from build123d import *

# Parameters (mm, degrees)
F1_DEPTH = 5
F9_R     = 1.5
F12_R    = 1.5
F15_R    = 1.5
F18_R    = 1.5
F21_R    = 1.5
F24_R    = 1.5
F28_R    = 1.5
F32_R    = 1.5
F31_R    = 1.5
F36_R    = 1.5


with BuildPart() as f1:
    # F0 (on Top) → F1 (new body, symmetric)
    with BuildSketch(Plane.XY):
        Polygon((-5, -5), (5, -5), (5, -1.9098300548), (0, 0), (-5, -1.9098300548), align=None)
        Polygon((0, 0), (5, -1.9098300548), (5, 1.9098300548), align=None)
        Polygon((-5, 1.9098300548), (-5, -1.9098300548), (0, 0), align=None)
        Polygon((0, 0), (5, 1.9098300548), (5, 5), (-5, 5), (-5, 1.9098300548), align=None)
    extrude(amount=F1_DEPTH, both=True)

    # F10: sweep along a path in F3
    with BuildLine(Plane(origin=(0, 0, 0), x_dir=(-0.7071067812, 0.7071067812, 0), z_dir=(0.7071067812, 0.7071067812, 0))) as f10_path:
        Line((-70.710678, 50), (70.710678, -50))
    # F9 (on line) → F10 (sweep)
    with BuildSketch(Plane(origin=(49.9999999161, -49.9999999161, 50), x_dir=(-0.8164965812, -0.4082482899, 0.4082482906), z_dir=(-0.5773502689, 0.5773502689, -0.5773502698))):
        Circle(F9_R)
    sweep(path=f10_path.line)

    # F13: sweep along a path in F3
    with BuildLine(Plane(origin=(0, 0, 0), x_dir=(-0.7071067812, 0.7071067812, 0), z_dir=(0.7071067812, 0.7071067812, 0))) as f13_path:
        Line((-70.710678, -50), (70.710678, 50))
    # F12 (on line) → F13 (sweep)
    with BuildSketch(Plane(origin=(49.9999999161, -49.9999999161, -50), x_dir=(-0.8164965812, -0.4082482899, -0.4082482906), z_dir=(-0.5773502689, 0.5773502689, 0.5773502698))):
        Circle(F12_R)
    sweep(path=f13_path.line)

    # F16: sweep along a path in F5
    with BuildLine(Plane(origin=(0, 0, 0), x_dir=(0.7071067812, 0.7071067812, 0), z_dir=(0.7071067812, -0.7071067812, 0))) as f16_path:
        Line((70.710678, -50), (-70.710678, 50))
    # F15 (on line) → F16 (sweep)
    with BuildSketch(Plane(origin=(-49.9999999161, -49.9999999161, 50), x_dir=(0.8164965812, -0.4082482899, 0.4082482906), z_dir=(-0.5773502689, -0.5773502689, 0.5773502698))):
        Circle(F15_R)
    sweep(path=f16_path.line)

    # F19: sweep along a path in F5
    with BuildLine(Plane(origin=(0, 0, 0), x_dir=(0.7071067812, 0.7071067812, 0), z_dir=(0.7071067812, -0.7071067812, 0))) as f19_path:
        Line((70.710678, 50), (-70.710678, -50))
    # F18 (on line) → F19 (sweep)
    with BuildSketch(Plane(origin=(-49.9999999161, -49.9999999161, -50), x_dir=(0.8164965812, -0.4082482899, -0.4082482906), z_dir=(-0.5773502689, -0.5773502689, -0.5773502698))):
        Circle(F18_R)
    sweep(path=f19_path.line)

    # F22: sweep along a path in F7
    with BuildLine(Plane.YZ) as f22_path:
        Line((-80.9016994, -30.9016994), (80.9016994, 30.9016994))
    # F21 (on line) → F22 (sweep)
    with BuildSketch(Plane(origin=(0, -80.9016994, -30.9016994), x_dir=(-1, 0, 0), z_dir=(0, 0.9341723591, 0.3568220895))):
        Circle(F21_R)
    sweep(path=f22_path.line)

    # F25: sweep along a path in F7
    with BuildLine(Plane.YZ) as f25_path:
        Line((-80.9016994, 30.9016994), (80.9016994, -30.9016994))
    # F24 (on line) → F25 (sweep)
    with BuildSketch(Plane(origin=(0, 80.9016994, -30.9016994), x_dir=(-1, 0, 0), z_dir=(0, 0.9341723591, -0.3568220895))):
        Circle(F24_R)
    sweep(path=f25_path.line)

    # F29: sweep along a path in F0
    with BuildLine(Plane.XY) as f29_path:
        Line((80.9016994, 30.9016994), (-80.9016994, -30.9016994))
    # F28 (on line) → F29 (sweep)
    with BuildSketch(Plane(origin=(80.9016994, 30.9016994, 0), x_dir=(0.3568220895, -0.9341723591, 0), z_dir=(-0.9341723591, -0.3568220895, 0))):
        Circle(F28_R)
    sweep(path=f29_path.line)

    # F33: sweep along a path in F0
    with BuildLine(Plane.XY) as f33_path:
        Line((-80.9016994, 30.9016994), (80.9016994, -30.9016994))
    # F32 (on line) → F33 (sweep)
    with BuildSketch(Plane(origin=(80.9016994, -30.9016994, 0), x_dir=(0.3568220895, 0.9341723591, 0), z_dir=(0.9341723591, -0.3568220895, 0))):
        Circle(F32_R)
    sweep(path=f33_path.line)

    # F34: sweep along a path in F6
    with BuildLine(Plane.XZ) as f34_path:
        Line((-30.9016994, -80.9016994), (30.9016994, 80.9016994))
    # F31 (on line) → F34 (sweep)
    with BuildSketch(Plane(origin=(30.9016994, 0, 80.9016994), x_dir=(0.9341723591, 0, -0.3568220895), z_dir=(0.3568220895, 0, 0.9341723591))):
        Circle(F31_R)
    sweep(path=f34_path.line)

    # F37: sweep along a path in F6
    with BuildLine(Plane.XZ) as f37_path:
        Line((-30.9016994, 80.9016994), (30.9016994, -80.9016994))
    # F36 (on line) → F37 (sweep)
    with BuildSketch(Plane(origin=(-30.9016994, 0, 80.9016994), x_dir=(0.9341723591, 0, 0.3568220895), z_dir=(0.3568220895, 0, -0.9341723591))):
        Circle(F36_R)
    sweep(path=f37_path.line)


solid = f1.part
The model under review builds one solid part; all positions refer to its coordinate system, in mm. Round coordinates to 2 decimals unless told otherwise and drop trailing zeros. Return JSON: item names as keys, results as strings.
1. Insertion check: P1, Ø12, axis at y = 63, z = 29, coming from the -X side; P2, Ø8, axis at y = -34, z = 42, coming from the -X side; P3, Ø12, axis at x = -13, z = 4, coming from the -Y side. Each pin has a flat end and moves straight along its axis. Give the tip position at first contact, or say it passes through.
Answer block:
{"P1": "stops at x = -1.5", "P2": "passes through", "P3": "stops at y = -11.79"}
2. Take a section at A-A (x = -11). State how many separate pieces and enclosed holes the cut face has, then the cut area to 3 significant figures.
Answer block:
{"separate pieces": "8", "enclosed holes": "0", "area": "104 mm²"}
3. For L1, parallel to Y at x = -14.5, z = 14.5; L2, parallel to X at y = -15, z = 14; L3, parallel to Y at x = 15, z = 41, list the stretches that pass through material, from the lowest coordinate up. Write a range as [from, to].
Answer block:
{"L1": "y = [-16.34, -12.66], [12.66, 16.34]", "L2": "x = [-16.12, -12.88], [12.88, 16.12]", "L3": "y = [-1.37, 1.37]"}
